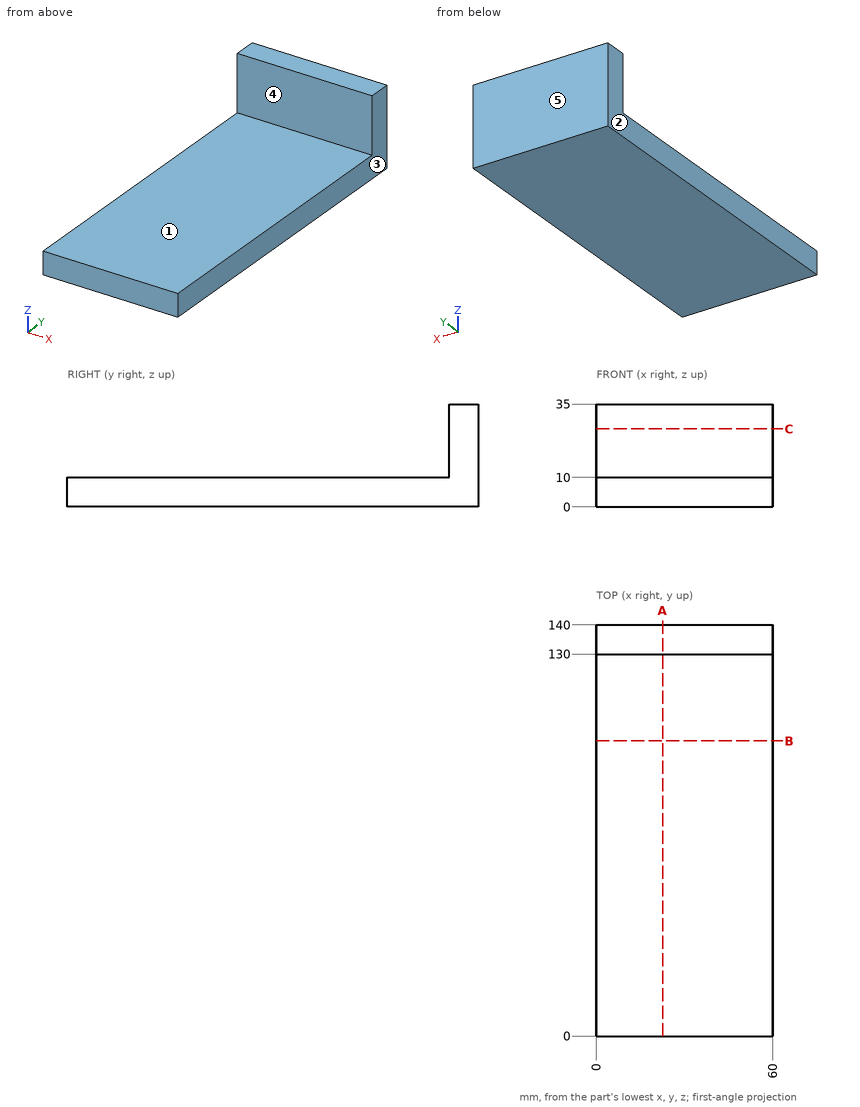
Geometry check sheet. Reference: drawing and pictorial views, mm from the part's lowest x, y, z. A direction names the side the tool comes from. Coordinates: 2 decimals unless noted, no trailing zeros. Write each loop counter-clockwise with the first axis right and the second up, starting at its lowest first coordinate (ties: lowest second). Pieces come first, ordered by that corner, then holes. Notation, with made-up numbers: (36.25, 62.5) -> (88.25, 62.5) arc R18 ccw to (88.25, 89.5) -> close; hole circle Ø8 at (79.25, -12.5). An arc over 180 degrees is marked (long way). Use a Markdown table: item, result.
1. Tool access check on the marked faces 4 and 5. Record the directions out of +Z, -Z, +X, -X, +Y, -Y that give a thin tool (end or side, any length) a straight path to the whole face; none if there is none.
Reported:
| item | result |
|---|---|
| face 4 | +Z, +X, -X, -Y |
| face 5 | +Z, -Z, +X, -X, +Y |
2. Sectioned sample at C-C (z = 26.5). Enter the section's corners in (x, y).
Reported:
| item | result |
|---|---|
| outline | (0, 130) -> (60, 130) -> (60, 140) -> (0, 140) -> close |
3. Scan lines: line 1 along Z through (x, y) = (24, 43); line 2 along Y through (x, z) = (24.5, 33). Record each from-to range of solid material in increasing order.
Reported:
| item | result |
|---|---|
| line 1 | z = 0 to 10 |
| line 2 | y = 130 to 140 |
4. Release check for a two-part mould opening along X. For the marked faces 1, 2 and 3 record: pulls with the +X half, pulls with the -X half, needs draft (parallel to the pull), parting line crosses it, or undercut.
Reported:
| item | result |
|---|---|
| face 1 | needs draft |
| face 2 | pulls with the -X half |
| face 3 | pulls with the +X half |
5. Sectioned sample at A-A (x = 22.5). Enter the section's corners in (y, z).
Reported:
| item | result |
|---|---|
| outline | (0, 0) -> (140, 0) -> (140, 35) -> (130, 35) -> (130, 10) -> (0, 10) -> close |
6. Sectioned sample at B-B (y = 100.5). Enter the section's corners in (x, z), plus the area to 3 significant figures.
Reported:
| item | result |
|---|---|
| outline | (0, 0) -> (60, 0) -> (60, 10) -> (0, 10) -> close |
| area | 600 mm2 |
7. Go/stop test with flat-tipped pins: pin 1 Ø5 at (x, y) = (41.5, 32) entering from +Z; pin 2 Ø12 at (y, z) = (58, 21.5) entering from +X. Record where each tip stops, or that it passes through.
Reported:
| item | result |
|---|---|
| pin 1 | stops at z = 10 |
| pin 2 | passes through |
